Verification items for this drawing (mm, ordinates from the low corner). A direction names the side the tool comes from. Round coordinates to 2 decimals unless told otherwise and drop trailing zeros. Order: outer loops, then holes, each group sorted by start corner. A loop starts at its lowest first (then second) coordinate and runs counter-clockwise, first axis right, second up. Notation, with made-up numbers: (29, 58) -> (48, 58) arc R21 cw to (48, 79) -> close; hole circle Ø3 at (85.25, 7.5). An arc over 180 degrees is marked (long way). Answer in a Markdown table with one row per item. Add a question column.
1. Sectioned sample at A-A, the plane x = 77.5. Record the boundary of the cut face in (y, z).
2. Material ranges on L1, parallel to Z at x = 77.5, y = 8; L2, parallel to X at y = 3.25, z = 17; L3, parallel to Z at x = 67.5, y = 6.5, recorded low to high. Write a range as from..to.
3. Sectioned sample at B-B, the plane z = 2.5. Record the boundary of the cut face in (x, y), then the cut area to 3 significant figures.
4. Access from +Z, -Z, +X, -X, +Y, -Y to the whole of each face (thin tool, end or side, straight path). Record for the marked faces 1, 2 and 3.
5. Sectioned sample at D-D, the plane x = 61. Record the boundary of the cut face in (y, z), then the cut area to 3 significant figures.
6. Depth check by flat-ended pin: P1, Ø2, axis at y = 5, z = 29, coming from the +X side; P2, Ø1.5, axis at x = 41.5, z = 17, coming from the -Y side; P3, Ø3.5, axis at x = 26, y = 3.5, coming from the -Z side; P4, Ø2, axis at x = 47.5, y = 3.5, coming from the +Z side. Enter the tip coordinate at first touch or a pass-through.
7. Sectioned sample at C-C, the plane z = 19. Record the boundary of the cut face in (x, y), then the cut area to 3 significant figures.
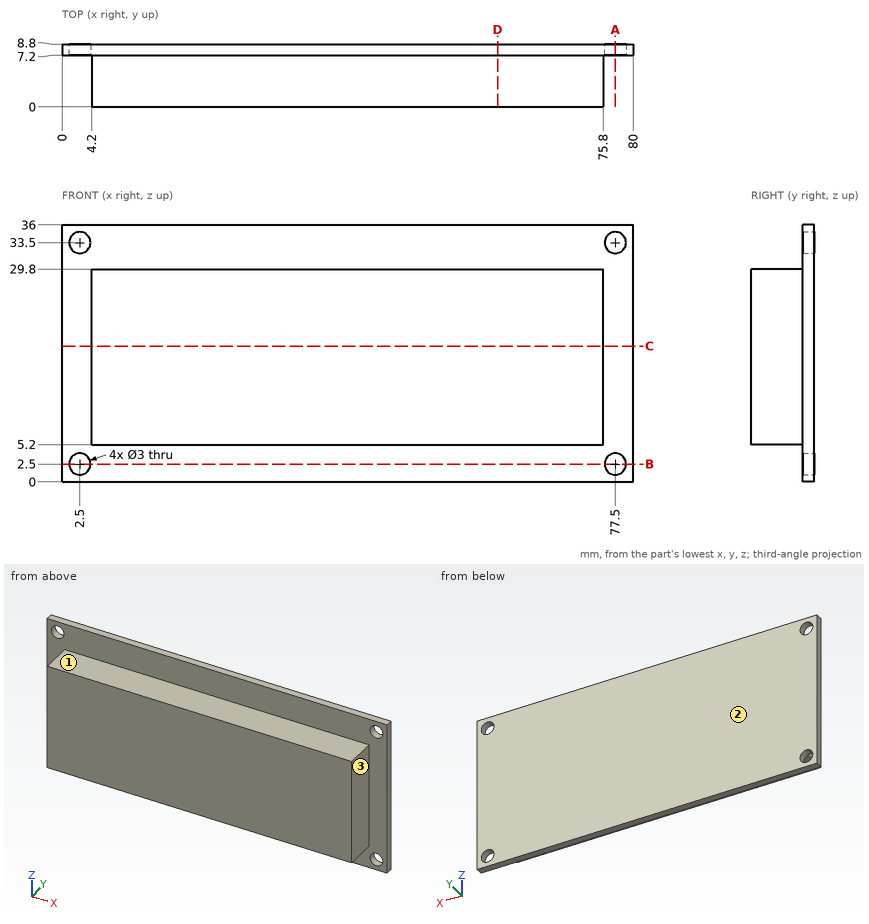
Answer key:
| question | item | result |
|---|---|---|
| 1 | outline | (7.2, 0) -> (8.8, 0) -> (8.8, 1) -> (7.2, 1) -> close; (7.2, 4) -> (8.8, 4) -> (8.8, 32) -> (7.2, 32) -> close; (7.2, 35) -> (8.8, 35) -> (8.8, 36) -> (7.2, 36) -> close |
| 2 | L1 | z = 0..1, 4..32, 35..36 |
| 2 | L2 | x = 4.2..75.8 |
| 2 | L3 | z = 5.2..29.8 |
| 3 | outline | (0, 7.2) -> (1, 7.2) -> (1, 8.8) -> (0, 8.8) -> close; (4, 7.2) -> (76, 7.2) -> (76, 8.8) -> (4, 8.8) -> close; (79, 7.2) -> (80, 7.2) -> (80, 8.8) -> (79, 8.8) -> close |
| 3 | area | 118 mm² |
| 4 | face 1 | +Z, +X, -X, -Y |
| 4 | face 2 | +Z, -Z, +X, -X, +Y |
| 4 | face 3 | +Z, -Z, +X, -Y |
| 5 | outline | (0, 5.2) -> (7.2, 5.2) -> (7.2, 0) -> (8.8, 0) -> (8.8, 36) -> (7.2, 36) -> (7.2, 29.8) -> (0, 29.8) -> close |
| 5 | area | 235 mm² |
| 6 | P1 | stops at x = 75.8 |
| 6 | P2 | stops at y = 0 |
| 6 | P3 | stops at z = 5.2 |
| 6 | P4 | stops at z = 29.8 |
| 7 | outline | (0, 7.2) -> (4.2, 7.2) -> (4.2, 0) -> (75.8, 0) -> (75.8, 7.2) -> (80, 7.2) -> (80, 8.8) -> (0, 8.8) -> close |
| 7 | area | 644 mm² |
